Build history of the part. All positions in model axes, mm. A direction names the side the tool comes from. Round coordinates to 2 decimals unless told otherwise and drop trailing zeros. Loops run counter-clockwise (first coordinate to the right, second up) from the corner with the lowest first, then second, coordinate; pieces in that order, holes last. Notation, with made-up numbers: (19, 9.5) - (74, 9.5) arc R26 ccw to (74, 38.5) - close; hole circle Ø5 at (76.5, 43). An arc over 180 degrees is marked (long way). Put each result on its own line as item: value. Start each with the question number.
from build123d import *

# Parameters (mm, degrees)
F1_DEPTH = 2133.6
F2_W     = 508
F2_H     = 1727.2
F3_DEPTH = 914.401


with BuildPart() as f1:
    # F0 (on Top) → F1 (new body)
    with BuildSketch(Plane.XY):
        Polygon((0, 609.6), (0, 0), (914.4, 0), (914.4, 25.4), (25.4, 25.4), (25.4, 609.6), align=None)
    extrude(amount=F1_DEPTH)

    # F2 (on face) → F3 (cut, through all)
    with BuildSketch(Plane(origin=(0, 0, 0), x_dir=(0, -1, 0), z_dir=(-1, 0, 0))):
        with Locations((-304.8, 1168.4)):
            Rectangle(F2_W, F2_H)
    extrude(amount=-F3_DEPTH, mode=Mode.SUBTRACT)


solid = f1.part
Item 1: Which spindle directions (+Z, -Z, +X, -X, +Y, -Y) get a long thin tool onto all of the face, cutting with end or side? Do faces 1 (the flat face through (0, 35, 1062)), 2 (the flat face through (25.4, 576, 746)). Say none if no direction does.
Item 2: Slice it at D-D (x = 511). Give the cut face in (y, z).
Item 3: Drill centre line: probe 1 along Y at (x, z) = (141, 972). Where is it in solid material? Low to high. Write a range as [from, to].
Item 4: Slice it at C-C (z = 279). Give the cut face in (x, y), plus the area to 3 significant figures.
Item 5: Slice it at A-A (y = 174). Give the cut face in (x, z), plus the area to 3 significant figures.
Item 6: Slice it at B-B (z = 1063). Give the cut face in (x, y).
Item 7: Drop flat-ended pins along their axis: pin 1 Ø4 at (y, z) = (340.5, 300.5) entering from +X; pin 2 Ø1.5 at (x, z) = (802, 728) entering from -Y; pin 3 Ø3 at (x, z) = (221, 974) entering from +Y. Give the stop position or say it passes through.
Computed values:
1. face 1: +Z, -Z, -X, +Y, -Y
1. face 2: +Z, -Z, +X, +Y
2. outline: (0, 0) - (25.4, 0) - (25.4, 2133.6) - (0, 2133.6) - close
3. probe 1: y = [0, 25.4]
4. outline: (0, 0) - (914.4, 0) - (914.4, 25.4) - (25.4, 25.4) - (25.4, 609.6) - (0, 609.6) - close
4. area: 38,100 mm^2
5. outline: (0, 0) - (25.4, 0) - (25.4, 304.8) - (0, 304.8) - close; (0, 2032) - (25.4, 2032) - (25.4, 2133.6) - (0, 2133.6) - close
5. area: 10,300 mm^2
6. outline: (0, 0) - (914.4, 0) - (914.4, 25.4) - (25.4, 25.4) - (25.4, 50.8) - (0, 50.8) - close; (0, 558.8) - (25.4, 558.8) - (25.4, 609.6) - (0, 609.6) - close
7. pin 1: stops at x = 25.4
7. pin 2: stops at y = 0
7. pin 3: stops at y = 25.4
